Study the drawing (mm; zero at the part's minimum x, y, z) and answer. Coordinates: 2 decimals unless noted, no trailing zeros. Write each loop counter-clockwise with the first axis right and the second up, starting at its lowest first coordinate (ties: lowest second). Pieces come first, ordered by that corner, then holes. Notation, with made-up numbers: M 78,60.5 L 110,60.5 A17 cw 110,65.5 Z; hole C 42.5,69 d2. An arc over 180 degrees is marked long. Answer as CSV lines item,"result". Start each with the question number.
(1) A cutting plane is placed at D-D on x = 43. Give the vertices of the cut face in (y, z), then the cut area to 3 significant figures.
(2) Flat-ended cylindrical pins translate along their axes: P1, Ø8, axis at x = 26, y = 62.5, coming from the -Z side; P2, Ø5, axis at x = 30.5, z = 6, coming from the -Y side; P3, Ø6, axis at x = 10.5, z = 3.5, coming from the -Y side. Find the tip coordinate at first contact, or state that the pin passes through.
(3) A cutting plane is placed at B-B on y = 27.5. Give the vertices of the cut face in (x, z).
(4) Find the intervals of material crossed by L1, parallel to Y at x = 25.4, z = 6.5; L2, parallel to X at y = 30, z = 2; L3, parallel to X at y = 34, z = 11, in increasing order. Write a range as [from, to].
(5) The mould has two halves that part along X. Classify the marked faces 1, 2, 3 and 4: released by +X, released by -X, zero draft, split by the parting line, or undercut.
(6) A cutting plane is placed at C-C on z = 2.5. Give the vertices of the cut face in (x, y).
(7) A cutting plane is placed at A-A on x = 25.4. Give the vertices of the cut face in (y, z).
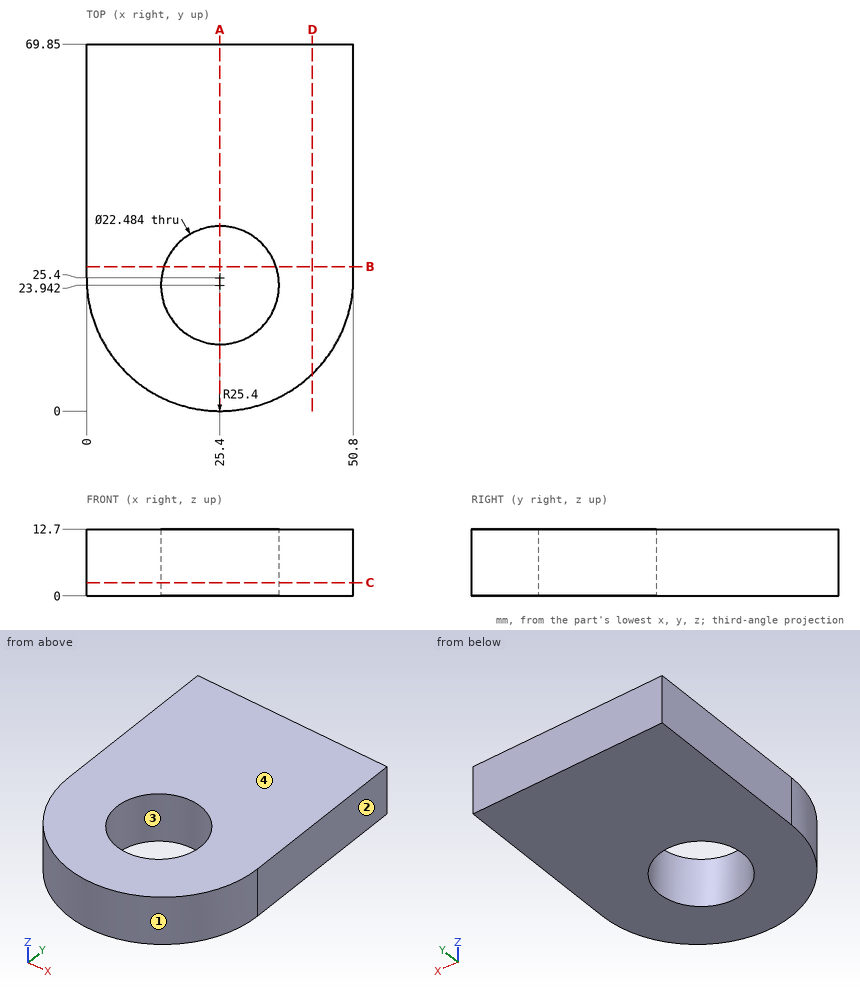
Here are the results:
1,outline,"M 7.09,0 L 69.85,0 L 69.85,12.7 L 7.09,12.7 Z"
1,area,"797 mm^2"
2,P1,"stops at z = 0"
2,P2,"stops at y = 0.13"
2,P3,"stops at y = 2.96"
3,outline,"M 0,0 L 14.74,0 L 14.74,12.7 L 0,12.7 Z; M 36.06,0 L 50.8,0 L 50.8,12.7 L 36.06,12.7 Z"
4,L1,"y = [0, 12.7], [35.18, 69.85]"
4,L2,"x = [0, 15.93], [34.87, 50.8]"
4,L3,"x = [0, 20.38], [30.42, 50.8]"
5,face 1,"split by the parting line"
5,face 2,"released by +X"
5,face 3,"undercut"
5,face 4,"zero draft"
6,outline,"M 0,25.4 A25.4 ccw 50.8,25.4 L 50.8,69.85 L 0,69.85 Z; hole C 25.4,23.94 d22.48"
7,outline,"M 0,0 L 12.7,0 L 12.7,12.7 L 0,12.7 Z; M 35.18,0 L 69.85,0 L 69.85,12.7 L 35.18,12.7 Z"
